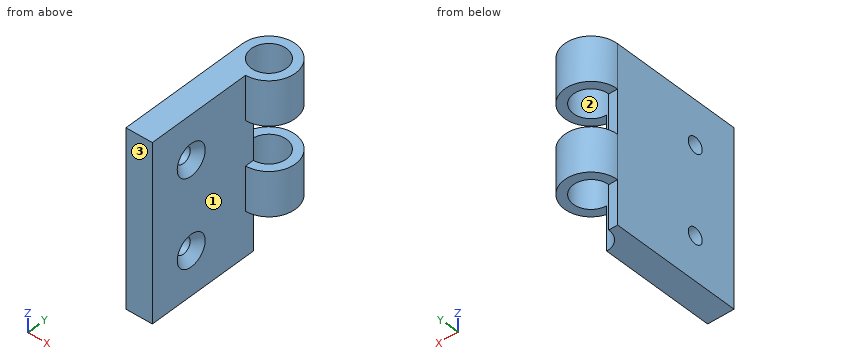
from build123d import *

# Parameters (mm, degrees)
SKETCH1_W                                            = 3
SKETCH1_H                                            = 15
BOSS_EXTRUDE1_DEPTH                                  = 20
SKETCH2_R                                            = 3
BOSS_EXTRUDE2_DEPTH                                  = 5
LPATTERN2_COUNT                                      = 2
LPATTERN2_PITCH                                      = 10
CUT_EXTRUDE1_DEPTH                                   = 26.709920264
CUT_EXTRUDE1_DEPTH_BACK                              = 26.709920264
SKETCH3_R                                            = 2
CSK_FOR_M1_6_COUNTERSUNK_FLAT_HEAD_SCREW_D           = 1.8
CSK_FOR_M1_6_COUNTERSUNK_FLAT_HEAD_SCREW_DEPTH       = 3
CSK_FOR_M1_6_COUNTERSUNK_FLAT_HEAD_SCREW_CSINK_D     = 3.6
CSK_FOR_M1_6_COUNTERSUNK_FLAT_HEAD_SCREW_CSINK_ANGLE = 90
CSK_FOR_M1_6_COUNTERSUNK_FLAT_HEAD_SCREW_TIP         = 0.540774557


with BuildPart() as part:
    # Sketch1 → Boss-Extrude1 (new body)
    with BuildSketch(Plane.XY):
        with Locations((1.5, -7.5)):
            Rectangle(SKETCH1_W, SKETCH1_H)
    extrude(amount=-BOSS_EXTRUDE1_DEPTH)

    # Sketch2 → Boss-Extrude2 (add)
    with BuildSketch(Plane.XY):
        with Locations((3, 0)):
            Circle(SKETCH2_R)
    boss_extrude2 = extrude(amount=-BOSS_EXTRUDE2_DEPTH)

    # LPattern2: Boss-Extrude2 ×2
    with Locations(*[(0, 0, -i * LPATTERN2_PITCH) for i in range(1, LPATTERN2_COUNT)]):
        add(boss_extrude2)

    # Sketch3 → Cut-Extrude1 (cut, two sides: drawn at the far end of the back side and taken through both)
    with BuildSketch(Plane.XY.offset(-CUT_EXTRUDE1_DEPTH_BACK)):
        with Locations((3, 0)):
            Circle(SKETCH3_R)
    extrude(amount=CUT_EXTRUDE1_DEPTH + CUT_EXTRUDE1_DEPTH_BACK, mode=Mode.SUBTRACT)

    # CSK for M1.6 Countersunk Flat Head Screw1
    with Locations(Plane(origin=(3, 0, 0), x_dir=(0, 0, -1), z_dir=(1, 0, 0))):
        with Locations((5, -10), (15, -10)):
            CounterSinkHole(CSK_FOR_M1_6_COUNTERSUNK_FLAT_HEAD_SCREW_D / 2, CSK_FOR_M1_6_COUNTERSUNK_FLAT_HEAD_SCREW_CSINK_D / 2, depth=CSK_FOR_M1_6_COUNTERSUNK_FLAT_HEAD_SCREW_DEPTH, counter_sink_angle=CSK_FOR_M1_6_COUNTERSUNK_FLAT_HEAD_SCREW_CSINK_ANGLE)
            with Locations((0, 0, -(CSK_FOR_M1_6_COUNTERSUNK_FLAT_HEAD_SCREW_DEPTH + CSK_FOR_M1_6_COUNTERSUNK_FLAT_HEAD_SCREW_TIP / 2))):  # 118° drill point
                Cone(0, CSK_FOR_M1_6_COUNTERSUNK_FLAT_HEAD_SCREW_D / 2, CSK_FOR_M1_6_COUNTERSUNK_FLAT_HEAD_SCREW_TIP, mode=Mode.SUBTRACT)


solid = part.part
The listing builds one solid part. Answer for the finished solid, in the listing's coordinates (mm). Face numbers are marked on the shaded views. Coordinates: 2 decimals unless noted, no trailing zeros. Loops run counter-clockwise (first coordinate to the right, second up) from the corner with the lowest first, then second, coordinate; pieces in that order, holes last.
1) Flat-ended cylindrical pins translate along their axes: pin 1 Ø1.8 at (x, y) = (4.5, 0.5) entering from -Z; pin 2 Ø0.5 at (x, z) = (0.5, -7) entering from +Y; pin 3 Ø2 at (x, z) = (3.5, -16.5) entering from +Y; pin 4 Ø3.5 at (x, y) = (3, 0) entering from -Z. Find the tip coordinate at first contact, or state that the pin passes through.
2) Find section D-D on x = 4.3. Write down the section's boundary in (y, z).
3) Find section B-B on z = -8. Write down the section's boundary in (x, y), then the cut area to 3 significant figures.
4) Find section A-A on y = -10. Write down the section's boundary in (x, z).
5) Determine the mould class of the marked faces 1, 2 and 3 for opening direction Y: pulls with the +Y half, pulls with the -Y half, needs draft (parallel to the pull), parting line crosses it, or undercut.
6) Find section C-C on y = 0.75. Write down the section's boundary in (x, z).
7) Find the intervals of material crossed by L1, parallel to Z at x = 1.6, y = -10; L2, parallel to Z at x = 5.15, y = 1.75; L3, parallel to Y at x = 0.6, z = -17, in increasing order.
Values:
1. pin 1: stops at z = -15
1. pin 2: stops at y = 0
1. pin 3: stops at y = -1.94
1. pin 4: passes through
2. outline: (-2.7, -15) - (-1.52, -15) - (-1.52, -10) - (-2.7, -10) - close; (-2.7, -5) - (-1.52, -5) - (-1.52, 0) - (-2.7, 0) - close; (1.52, -15) - (2.7, -15) - (2.7, -10) - (1.52, -10) - close; (1.52, -5) - (2.7, -5) - (2.7, 0) - (1.52, 0) - close
3. outline: (0, -15) - (3, -15) - (3, -2) arc R2 cw to (1, 0) - (0, 0) - close
3. area: 41.9 mm2
4. outline: (0, -20) - (3, -20) - (3, -16.8) - (2.1, -15.9) - (0, -15.9) - close; (0, -14.1) - (2.1, -14.1) - (3, -13.2) - (3, -6.8) - (2.1, -5.9) - (0, -5.9) - close; (0, -4.1) - (2.1, -4.1) - (3, -3.2) - (3, 0) - (0, 0) - close
5. face 1: needs draft
5. face 2: undercut
5. face 3: pulls with the -Y half
6. outline: (0.1, -15) - (1.15, -15) - (1.15, -10) - (0.1, -10) - close; (0.1, -5) - (1.15, -5) - (1.15, 0) - (0.1, 0) - close; (4.85, -15) - (5.9, -15) - (5.9, -10) - (4.85, -10) - close; (4.85, -5) - (5.9, -5) - (5.9, 0) - (4.85, 0) - close
7. L1: z = -20 to -15.9, -14.1 to -5.9, -4.1 to 0
7. L2: z = -15 to -10, -5 to 0
7. L3: y = -15 to 0
